Source: CAD feature listing. Evaluate the final solid. Frame: model axes, mm. Face numbers are marked on the shaded views. A direction names the side the tool comes from. Give positions to 0.01 mm unless a question says otherwise; leave off trailing zeros. Write each loop counter-clockwise with the first axis right and the second up, starting at its lowest first coordinate (ties: lowest second). Pieces come first, ordered by that corner, then holes. Notation, with made-up numbers: (71.5, 55) -> (99.5, 55) arc R33 ccw to (99.5, 89) -> close; hole circle Ø3 at (30.25, 67.25). An arc over 180 degrees is marked (long way). Answer as a JSON object with one key per item and string values. Group by question number.
Item 1: Pull-direction query (Y, two-part tool) for the marked faces 6, 7 and 8; classes: pulls with the +Y half, pulls with the -Y half, needs draft (parallel to the pull), parting line crosses it, or undercut.
Item 2: First-contact query: pin 1 Ø10 at (x, z) = (-8.5, 10.5) entering from +Y; pin 2 Ø13.5 at (x, y) = (-5.5, -8.5) entering from -Z; pin 3 Ø2 at (x, y) = (-12, -1.5) entering from +Z. Flat tips, straight axial feed; report the tip coordinate or a pass-through.
Item 3: Section query C-C on x = -12. Give the number of separate pieces and of enclosed holes in the cut face, plus the area to 3 significant figures.
Item 4: Section query A-A on y = -11. Return the cut outline in (x, z).
Item 5: Section query B-B on z = -20. Return the cut outline in (x, y).
Item 6: Ray query, probe 1 along X at (y, z) = (3, 1.5); probe 2 along Z at (x, y) = (7.75, 12.7); probe 3 along X at (y, z) = (-18.5, 19). Return the intervals inside material, ascending. Write a range as from..to.
Item 7: Access query for the marked faces 1, 2, 3, 4 and 5. Directions: +Z, -Z, +X, -X, +Y, -Y. A direction counts if a zero-diameter tool reaches every point of the face in a straight line with its end or side. Return the directions, or none.
Item 8: Section query D-D on y = 12.7. Return the cut outline in (x, z), plus the area to 3 significant figures.
from build123d import *

# Parameters (mm, degrees)
F0_W      = 50.8
F0_H      = 50.8
F1_DEPTH  = 25.4
F3_DEPTH  = 25.4
F4_R      = 3.175
F5_DEPTH  = 50.801
F6_W      = 6.35
F6_H      = 29.9948125449
F6_H_2    = 12.7
F7_DEPTH  = 50.801
F8_R      = 3.175
F9_DEPTH  = 6.35
F10_DEPTH = 6.35
F11_DEPTH = 1.5875


# Not quite as in the source:
# - a feature names something its author has since deleted; it is built from what else it names


with BuildPart() as f1:
    # F0 (on Front) → F1 (new body, symmetric)
    with BuildSketch(Plane.XZ):
        with Locations((-1.9110422581, 1.9712704602)):
            Rectangle(F0_W, F0_H)
    extrude(amount=F1_DEPTH, both=True)

    # F2 (on face) → F3 (cut)
    with BuildSketch(Plane(origin=(0, 0, -23.4287295398), x_dir=(1, 0, 0), z_dir=(0, 0, -1))):
        with BuildLine():
            Line((-6.6735422581, -6.4520295568), (-6.6735422581, 0))
            ThreePointArc((-6.6735422581, 0), (-8.2610422581, 12.4983610621), (-9.8485422581, 0))
            Line((-9.8485422581, 0), (-9.8485422581, -6.4520295568))
            ThreePointArc((-9.8485422581, -6.4520295568), (-8.2610422581, -6.5516389379), (-6.6735422581, -6.4520295568))
        make_face()
        with BuildLine():
            Line((-6.6735422581, -25.4), (-6.6735422581, -6.4520295568))
            ThreePointArc((-6.6735422581, -6.4520295568), (-8.2610422581, -6.5516389379), (-9.8485422581, -6.4520295568))
            Line((-9.8485422581, -6.4520295568), (-9.8485422581, -25.4))
            Line((-9.8485422581, -25.4), (-6.6735422581, -25.4))
        make_face()
    extrude(amount=-F3_DEPTH, mode=Mode.SUBTRACT)

    # F4 (on face) → F5 (cut, through all)
    with BuildSketch(Plane.YZ.offset(23.4889577419)):
        with BuildLine():
            Line((-25.4, 27.3712704602), (-25.4, 14.6712704602))
            ThreePointArc((-25.4, 14.6712704602), (-21.6802561342, 23.6515265681), (-12.7000000372, 27.3712704602))
            Line((-12.7000000372, 27.3712704602), (-25.4, 27.3712704602))
        make_face()
        with BuildLine():
            Line((0, 14.6712704602), (0, 1.9712704602))
            Line((0, 1.9712704602), (25.4, 1.9712704602))
            Line((25.4, 1.9712704602), (25.4, 27.3712704602))
            Line((25.4, 27.3712704602), (-12.7000000372, 27.3712704602))
            ThreePointArc((-12.7000000372, 27.3712704602), (-3.7197438921, 23.6515265944), (0, 14.6712704602))
        make_face()
        with Locations((-12.7, 14.6712704602)):
            Circle(F4_R)
        with Locations((12.7, -10.7287295398)):
            Circle(F4_R)
    extrude(amount=-F5_DEPTH, mode=Mode.SUBTRACT)

    # F6 (on face) → F7 (cut, through all)
    with BuildSketch(Plane.XZ.offset(25.4)):
        with Locations((7.6139577419, 29.6686767327)):
            Rectangle(F6_W, F6_H)
        with Locations((7.6139577419, 8.3212704602)):
            Rectangle(F6_W, F6_H_2)
    extrude(amount=-F7_DEPTH, mode=Mode.SUBTRACT)

    # F8 (on face) → F9 (cut)
    with BuildSketch(Plane(origin=(-27.3110422581, 0, 0), x_dir=(0, -1, 0), z_dir=(-1, 0, 0))):
        Polygon((9.0338257906, 21.0212704602), (5.3676515813, 14.6712704602), (9.0338257906, 8.3212704602), (16.3661742094, 8.3212704602), (20.0323484187, 14.6712704602), (16.3661742094, 21.0212704602), align=None)
        with Locations((12.7, 14.6712704602)):
            Circle(F8_R, mode=Mode.SUBTRACT)
    extrude(amount=-F9_DEPTH, mode=Mode.SUBTRACT)

    # F4 (on face) → F10 (cut)
    with BuildSketch(Plane.YZ.offset(23.4889577419)):
        Polygon((16.4270880107, -17.0431692056), (20.0320091667, -10.6581964733), (16.3049211559, -4.3437568074), (8.9729119893, -4.414289874), (5.3679908333, -10.7992626063), (9.0950788441, -17.1137022722), align=None)
        with Locations((12.7, -10.7287295398)):
            Circle(F4_R, mode=Mode.SUBTRACT)
    extrude(amount=-F10_DEPTH, mode=Mode.SUBTRACT)

    # F2 (on face) → F11 (cut)
    with BuildSketch(Plane(origin=(0, 0, -23.4287295398), x_dir=(1, 0, 0), z_dir=(0, 0, -1))):
        with BuildLine():
            ThreePointArc((-9.8485422581, 0), (-8.2610422581, 12.4983610621), (-6.6735422581, 0))
            Line((-6.6735422581, 0), (-6.6735422581, -6.4520295568))
            ThreePointArc((-6.6735422581, -6.4520295568), (1.2639577419, -2.2518993505), (4.4389577419, 6.1483610621))
            ThreePointArc((4.4389577419, 6.1483610621), (-16.6613026708, 15.6733610621), (-9.8485422581, -6.4520295568))
            Line((-9.8485422581, -6.4520295568), (-9.8485422581, 0))
        make_face()
    extrude(amount=-F11_DEPTH, mode=Mode.SUBTRACT)


solid = f1.part
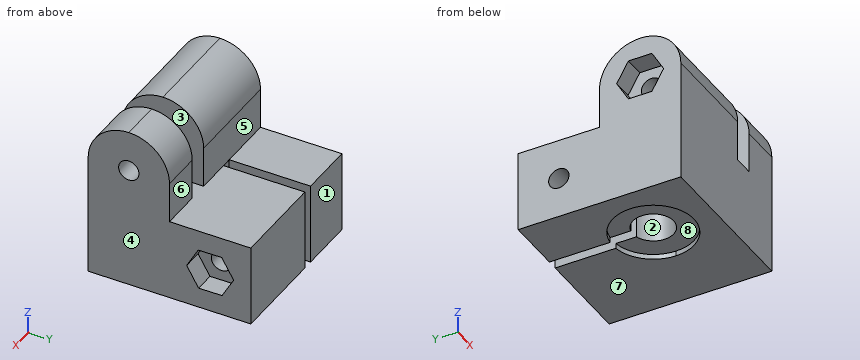
Worked answers:
{
 "1": {"face 6": "pulls with the +Y half", "face 7": "needs draft", "face 8": "undercut"},
 "2": {"pin 1": "y = 0", "pin 2": "z = -21.84", "pin 3": "z = 22.24"},
 "3": {"separate pieces": "1", "enclosed holes": "2", "area": "1,520 mm^2"},
 "4": {"outline": "(-27.31, -23.43) -> (-20, -23.43) -> (-20, -21.84) -> (-12.36, -21.84) -> (-12.36, 1.97) -> (-4.16, 1.97) -> (-4.16, -21.84) -> (3.48, -21.84) -> (3.48, -23.43) -> (23.49, -23.43) -> (23.49, 11.99) -> (10.79, 11.99) -> (10.79, 1.97) -> (4.44, 1.97) -> (4.44, 11.99) -> (-20.96, 11.99) -> (-20.96, 8.32) -> (-27.31, 8.32) -> close; (-27.31, 21.02) -> (-20.96, 21.02) -> (-20.96, 17.35) -> (4.44, 17.35) -> (4.44, 27.26) -> (-27.31, 27.26) -> close; (10.79, 17.35) -> (23.49, 17.35) -> (23.49, 27.26) -> (10.79, 27.26) -> close"},
 "5": {"outline": "(-27.31, -25.4) -> (23.49, -25.4) -> (23.49, 25.4) -> (-6.67, 25.4) -> (-6.67, 0) arc R6.35 cw (long way) to (-9.85, 0) -> (-9.85, 25.4) -> (-27.31, 25.4) -> close"},
 "6": {"probe 1": "-27.31..-9.85, -6.67..23.49", "probe 2": "-23.43..-13.9, -7.55..1.97", "probe 3": "-27.31..4.44, 10.79..23.49"},
 "7": {"face 1": "+Z, -Z, +X, -X, +Y", "face 2": "-Z", "face 3": "+Z, +Y, -Y", "face 4": "+Z, -Z, +X, +Y, -Y", "face 5": "+Z, +X, -X, +Y"},
 "8": {"outline": "(-27.31, -23.43) -> (-9.85, -23.43) -> (-9.85, -13.9) -> (-27.31, -13.9) -> close; (-27.31, -7.55) -> (-9.85, -7.55) -> (-9.85, 1.97) -> (-27.31, 1.97) -> close; (-6.67, -23.43) -> (23.49, -23.43) -> (23.49, -17.08) -> (17.14, -17.08) -> (17.14, -13.9) -> (-6.67, -13.9) -> close; (-6.67, -7.55) -> (17.14, -7.55) -> (17.14, -4.38) -> (23.49, -4.38) -> (23.49, 1.97) -> (-6.67, 1.97) -> close", "area": "867 mm^2"}
}
